Autodesk Inventor part; units mm, degrees
ref_plane "YZ Plane" through (0, 0, 0) normal (1, 0, 0) x (0, 1, 0)
ref_plane "XZ Plane" through (0, 0, 0) normal (0, 1, 0) x (-1, 0, 0)
ref_plane "XY Plane" through (0, 0, 0) normal (0, 0, 1) x (1, 0, 0)
sketch "Sketch1" plane through (0, 0, 0) normal (0, 0, 1) x (1, 0, 0)
  line L0 (-222.25, -238.125) -> (222.25, -238.125)
  line L1 (222.25, -238.125) -> (222.25, 238.125)
  line L2 (222.25, 238.125) -> (-222.25, 238.125)
  line L3 (-222.25, 238.125) -> (-222.25, -238.125)
  line L4 (-222.25, -238.125) -> (222.25, 238.125) construction
  line L5 (222.25, -238.125) -> (-222.25, 238.125) construction
  point P0 (0, 0)
  dimension "d0" = 444.5
  dimension "d1" = 476.25
extrude "Extrusion1" add sketch "Sketch1" along normal blind 3.175
sketch "Sketch3" plane through (0, 0, 3.175) normal (0, 0, 1) x (1, 0, 0)
  line L0 (-222.25, -238.125) -> (222.25, -238.125) construction
  line L1 (222.25, -238.125) -> (222.25, -161.925) construction
  line L2 (222.25, -238.125) -> (222.25, 238.125) construction
  line L3 (222.25, -161.925) -> (101.6, -161.925) construction
  line L4 (63.5, -212.725) -> (139.7, -212.725)
  line L5 (139.7, -212.725) -> (139.7, -111.125)
  line L6 (139.7, -111.125) -> (63.5, -111.125)
  line L7 (63.5, -111.125) -> (63.5, -212.725)
  line L8 (63.5, -212.725) -> (139.7, -111.125) construction
  line L9 (139.7, -212.725) -> (63.5, -111.125) construction
  point P0 (0, 0)
  dimension "d10" = 76.2
  dimension "d11" = 120.65
  dimension "d12" = 76.2
  dimension "d13" = 101.6
extrude "Extrusion3" cut sketch "Sketch3" against normal through all
sketch "Sketch4" plane through (0, 0, 3.175) normal (0, 0, 1) x (1, 0, 0)
  line L0 (222.25, -238.125) -> (222.25, 238.125) construction
  line L1 (222.25, 238.125) -> (222.25, 161.925) construction
  line L2 (222.25, 161.925) -> (101.6, 161.925) construction
  line L3 (63.5, 111.125) -> (139.7, 111.125)
  line L4 (139.7, 111.125) -> (139.7, 212.725)
  line L5 (139.7, 212.725) -> (63.5, 212.725)
  line L6 (63.5, 212.725) -> (63.5, 111.125)
  line L7 (63.5, 111.125) -> (139.7, 212.725) construction
  line L8 (139.7, 111.125) -> (63.5, 212.725) construction
  point P0 (0, 0)
  dimension "d16" = 76.2
  dimension "d17" = 120.65
  dimension "d18" = 76.2
  dimension "d19" = 101.6
extrude "Extrusion4" cut sketch "Sketch4" against normal through all
sketch "Sketch5" plane through (0, 0, 0) normal (0, 0, -1) x (-1, 0, 0)
  line L0 (-222.25, -238.125) -> (-222.25, 238.125)
  line L1 (-222.25, -238.125) -> (-158.75, -238.125)
  line L2 (-158.75, -238.125) -> (-158.75, -212.725)
  line L3 (-158.75, -212.725) -> (-222.25, -212.725)
  line L4 (-222.25, -212.725) -> (-222.25, -238.125)
  point P0 (0, 0)
  dimension "d22" = 63.5
  dimension "d23" = 25.4
extrude "Extrusion5" cut sketch "Sketch5" against normal through all
sketch "Sketch6" plane through (0, 0, 0) normal (0, 0, -1) x (-1, 0, 0)
  line L0 (-222.25, 238.125) -> (-158.75, 238.125)
  line L1 (-158.75, 238.125) -> (-158.75, 212.725)
  line L2 (-158.75, 212.725) -> (-222.25, 212.725)
  line L3 (-222.25, 212.725) -> (-222.25, 238.125)
  point P0 (0, 0)
  dimension "d26" = 63.5
  dimension "d27" = 25.4
extrude "Extrusion6" cut sketch "Sketch6" against normal through all
sketch "Sketch7" plane through (0, 0, 0) normal (0, 0, -1) x (-1, 0, 0)
  line L0 (-158.75, 238.125) -> (222.25, 238.125)
  line L1 (222.25, 238.125) -> (137.16, 238.125)
  line L2 (137.16, 238.125) -> (137.16, 212.725)
  line L3 (137.16, 212.725) -> (196.85, 212.725)
  line L4 (222.25, 217.4302) -> (222.25, 238.125)
  line L5 (222.25, 238.125) -> (187.6675, 238.125)
  line L6 (196.85, 212.725) -> (196.85, 178.435)
  line L7 (196.85, 178.435) -> (222.25, 178.435)
  line L8 (222.25, 178.435) -> (222.25, 238.125)
  point P0 (0, 0)
  dimension "d31" = 25.4
  dimension "d32" = 25.4
  dimension "d36" = 59.69
  dimension "d37" = 85.09
extrude "Extrusion7" cut sketch "Sketch7" against normal through all
sketch "Sketch8" plane through (0, 0, 0) normal (0, 0, -1) x (-1, 0, 0)
  line L0 (222.25, -238.125) -> (-158.75, -238.125)
  line L1 (222.25, -238.125) -> (196.85, -238.125)
  line L2 (196.85, -212.725) -> (196.85, -178.435)
  line L3 (196.85, -178.435) -> (222.25, -178.435)
  line L4 (222.25, -178.435) -> (222.25, -238.125)
  line L5 (222.25, -238.125) -> (137.16, -238.125)
  line L6 (137.16, -238.125) -> (137.16, -212.725)
  line L7 (137.16, -212.725) -> (196.85, -212.725)
  line L8 (222.25, -212.725) -> (222.25, -238.125)
  point P0 (0, 0)
  dimension "d38" = 25.4
  dimension "d39" = 59.69
  dimension "d40" = 85.09
  dimension "d41" = 25.4
extrude "Extrusion8" cut sketch "Sketch8" against normal through all
sketch "Sketch9" plane through (0, 0, 0) normal (0, 0, -1) x (-1, 0, 0)
  line L0 (-158.75, 212.725) -> (-158.75, 238.125) construction
  line L1 (-158.75, 225.425) -> (6.35, 225.425) construction
  line L2 (-50.8, 238.125) -> (63.5, 238.125)
  line L3 (63.5, 238.125) -> (63.5, 212.725)
  line L4 (63.5, 212.725) -> (-50.8, 212.725)
  line L5 (-50.8, 212.725) -> (-50.8, 238.125)
  line L6 (-50.8, 238.125) -> (63.5, 212.725) construction
  line L7 (63.5, 238.125) -> (-50.8, 212.725) construction
  line L8 (-158.75, -238.125) -> (-158.75, -212.725) construction
  line L9 (-158.75, -225.425) -> (6.35, -225.425) construction
  line L10 (-50.8, -212.725) -> (63.5, -212.725)
  line L11 (63.5, -212.725) -> (63.5, -238.125)
  line L12 (63.5, -238.125) -> (-50.8, -238.125)
  line L13 (-50.8, -238.125) -> (-50.8, -212.725)
  line L14 (-50.8, -212.725) -> (63.5, -238.125) construction
  line L15 (63.5, -212.725) -> (-50.8, -238.125) construction
  point P0 (0, 0)
  dimension "d44" = 165.1
  dimension "d45" = 114.3
  dimension "d46" = 25.4
  dimension "d47" = 165.1
  dimension "d48" = 114.3
  dimension "d49" = 25.4
extrude "Extrusion9" cut sketch "Sketch9" against normal through all
properties part number "Bellypan"
Here's how the part is built. I have some questions about the finished solid (model axes, mm). Coordinates: 2 decimals unless noted, no trailing zeros. Loops run counter-clockwise (first coordinate to the right, second up) from the corner with the lowest first, then second, coordinate; pieces in that order, holes last. Notation, with made-up numbers: (71.5, -33.5) - (127.5, -33.5) arc R26 cw to (127.5, 1.5) - close; hole circle Ø2 at (57, 45.5). An arc over 180 degrees is marked (long way). Return JSON: item names as keys, results as strings. Group by question number.
Item 1: If we section it at A-A on y = -135: Write out the boundary of the cut face in (x, z) (3 decimals), and give its area (3 significant figures).
Item 2: If we section it at D-D on x = -163: Write out the boundary of the cut face in (y, z) (3 decimals).
Item 3: Will these pins go through, and if not, where does the flat tip stop? P1, Ø1.6, axis at x = -169.5, z = 2.5, coming from the +Y side (3 decimals); P2, Ø1, axis at y = -196.5, z = 1.5, coming from the -X side; P3, Ø1, axis at y = 222.5, z = 1.5, coming from the -X side.
Item 4: I need wall thicknesses on line 1 (Y direction, x = 119, z = 2.4) (3 decimals); line 2 (X direction, y = -150, z = 2.75); line 3 (Y direction, x = -202.5, z = 0.2) (3 decimals). Which ranges of each line are inside material? Lowest first, please. Write a range as from..to.
Item 5: If we section it at B-B on z = 1.7: State how many separate pieces and enclosed holes the cut face has, and give its area (3 significant figures).
Item 6: If we section it at C-C on y = 205.5: Write out the boundary of the cut face in (x, z) (3 decimals), and give its area (3 significant figures).
Calculated:
{
 "1": {"outline": "(-222.25, 0) - (63.5, 0) - (63.5, 3.175) - (-222.25, 3.175) - close; (139.7, 0) - (222.25, 0) - (222.25, 3.175) - (139.7, 3.175) - close", "area": "1,170 mm^2"},
 "2": {"outline": "(-212.725, 0) - (212.725, 0) - (212.725, 3.175) - (-212.725, 3.175) - close"},
 "3": {"P1": "stops at y = 212.725", "P2": "stops at x = -196.85", "P3": "stops at x = -137.16"},
 "4": {"line 1": "y = -238.125..-212.725, -111.125..111.125, 212.725..238.125", "line 2": "x = -222.25..63.5, 139.7..222.25", "line 3": "y = -178.435..178.435"},
 "5": {"separate pieces": "1", "enclosed holes": "2", "area": "181,000 mm^2"},
 "6": {"outline": "(-196.85, 0) - (63.5, 0) - (63.5, 3.175) - (-196.85, 3.175) - close; (139.7, 0) - (222.25, 0) - (222.25, 3.175) - (139.7, 3.175) - close", "area": "1,090 mm^2"}
}
